Part model, mm, in its own coordinate system. Face numbers are marked on the shaded views. A direction names the side the tool comes from. Coordinates: 2 decimals unless noted, no trailing zeros. Order: outer loops, then holes, each group sorted by start corner. A loop starts at its lowest first (then second) coordinate and runs counter-clockwise, first axis right, second up. Notation, with made-up numbers: M 62,-28.5 L 117,-28.5 A19 ccw 117,4.5 Z; hole C 66.25,41.25 d3. An arc over 180 degrees is marked long. Answer in a Markdown table with one row per item. Add a question column.
from build123d import *

# Parameters (mm, degrees)
SKETCH1_W           = 30
SKETCH1_H           = 15
BOSS_EXTRUDE1_DEPTH = 15
SKETCH2_R           = 7.5
CUT_EXTRUDE1_DEPTH  = 15
CUT_EXTRUDE2_REACH  = 5
SKETCH3_R           = 2


with BuildPart() as part:
    # Sketch1 → Boss-Extrude1 (new body)
    with BuildSketch(Plane.XY):
        Rectangle(SKETCH1_W, SKETCH1_H)
    extrude(amount=BOSS_EXTRUDE1_DEPTH)

    # Sketch2 → Cut-Extrude1 (cut)
    with BuildSketch(Plane.XZ.offset(7.5)):
        with Locations((0, 15)):
            Circle(SKETCH2_R)
        with BuildLine():
            Line((-15, 12), (-9, 12))
            Line((-9, 12), (-8.485281374, 12))
            ThreePointArc((-8.485281374, 12), (0, 6), (8.485281374, 12))
            Line((8.485281374, 12), (9, 12))
            Line((9, 12), (15, 12))
            Line((15, 12), (15, 0))
            Line((15, 0), (11, 0))
            Line((11, 0), (-11, 0))
            Line((-11, 0), (-15, 0))
            Line((-15, 0), (-15, 12))
        make_face()
    extrude(amount=-CUT_EXTRUDE1_DEPTH, mode=Mode.SUBTRACT)

    # Sketch3 → Cut-Extrude2 (cut, up to next)
    with BuildSketch(Plane(origin=(0, 0, 12), x_dir=(-1, 0, 0), z_dir=(0, 0, -1)), mode=Mode.PRIVATE) as cut_extrude2_sk1:
        with Locations((11.3, -4.5)):
            Circle(SKETCH3_R)
    cut_extrude2_tool1 = extrude(cut_extrude2_sk1.sketch, amount=-CUT_EXTRUDE2_REACH, mode=Mode.PRIVATE) & part.part
    add(cut_extrude2_tool1.solids().sort_by_distance((-11.3, -4.5, 12))[0], mode=Mode.SUBTRACT)
    # Sketch3 → Cut-Extrude2 (cut, up to next)
    with BuildSketch(Plane(origin=(0, 0, 12), x_dir=(-1, 0, 0), z_dir=(0, 0, -1)), mode=Mode.PRIVATE) as cut_extrude2_sk2:
        with Locations((11.3, 4.5)):
            Circle(SKETCH3_R)
    cut_extrude2_tool2 = extrude(cut_extrude2_sk2.sketch, amount=-CUT_EXTRUDE2_REACH, mode=Mode.PRIVATE) & part.part
    add(cut_extrude2_tool2.solids().sort_by_distance((-11.3, 4.5, 12))[0], mode=Mode.SUBTRACT)
    # Sketch3 → Cut-Extrude2 (cut, up to next)
    with BuildSketch(Plane(origin=(0, 0, 12), x_dir=(-1, 0, 0), z_dir=(0, 0, -1)), mode=Mode.PRIVATE) as cut_extrude2_sk3:
        with Locations((-11.3, 4.5)):
            Circle(SKETCH3_R)
    cut_extrude2_tool3 = extrude(cut_extrude2_sk3.sketch, amount=-CUT_EXTRUDE2_REACH, mode=Mode.PRIVATE) & part.part
    add(cut_extrude2_tool3.solids().sort_by_distance((11.3, 4.5, 12))[0], mode=Mode.SUBTRACT)
    # Sketch3 → Cut-Extrude2 (cut, up to next)
    with BuildSketch(Plane(origin=(0, 0, 12), x_dir=(-1, 0, 0), z_dir=(0, 0, -1)), mode=Mode.PRIVATE) as cut_extrude2_sk4:
        with Locations((-11.3, -4.5)):
            Circle(SKETCH3_R)
    cut_extrude2_tool4 = extrude(cut_extrude2_sk4.sketch, amount=-CUT_EXTRUDE2_REACH, mode=Mode.PRIVATE) & part.part
    add(cut_extrude2_tool4.solids().sort_by_distance((11.3, -4.5, 12))[0], mode=Mode.SUBTRACT)


solid = part.part
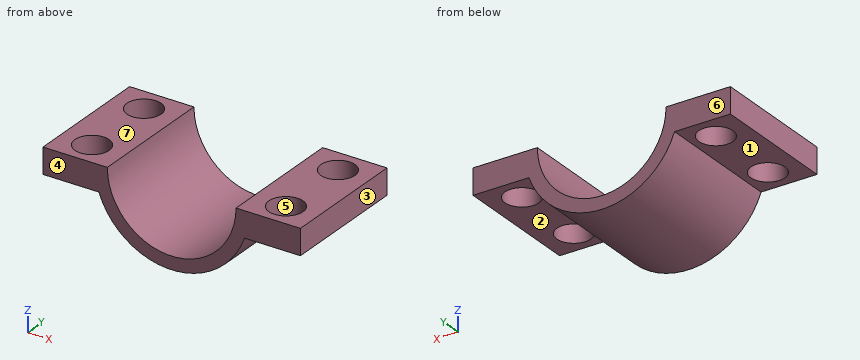
(1) Wall check: line 1 (Y direction, x = -11.3, z = 12.8); line 2 (Y direction, x = 10.25, z = 12.5); line 3 (X direction, y = -3, z = 12.5). Give the ranges that are in metal, low to high.
(2) Slice it at D-D (y = -1). List the corners of the cut face in (x, z).
(3) Drop flat-ended pins along their axis: P1, Ø4.5, axis at x = -11.3, y = 4.5, coming from the -Z side; P2, Ø1, axis at y = -2, z = 11, coming from the -X side; P3, Ø6.5, axis at x = -11.3, y = -4.5, coming from the -Z side. Give the stop position or say it passes through.
(4) 3-axis set-ups, long thin cutter, end or side, ignore diameter. For the marked faces 1, 2 and 3: which of +Z, -Z, +X, -X, +Y, -Y reach the whole face in a straight line?
(5) Slice it at A-A (x = -11.3). List the corners of the cut face in (y, z).
(6) Slice it at B-B (y = -4.5). List the corners of the cut face in (x, z), and give its area (3 significant figures).
(7) Pull direction Y, two halves, no side cores. Call the marked faces 4, 5, 6 and 7: pulls with the +Y half, pulls with the -Y half, needs draft (parallel to the pull), parting line crosses it, or undercut.
(8) Slice it at C-C (z = 8.5). List the corners of the cut face in (x, y), and give its area (3 significant figures).
Computed:
| question | item | result |
|---|---|---|
| 1 | line 1 | y = -7.5 to -6.5, -2.5 to 2.5, 6.5 to 7.5 |
| 1 | line 2 | y = -7.5 to -6.2, -2.8 to 2.8, 6.2 to 7.5 |
| 1 | line 3 | x = -15 to -12.62, -9.98 to -7.07, 7.07 to 9.98, 12.62 to 15 |
| 2 | outline | M -15,12 L -8.49,12 A9 ccw 8.49,12 L 15,12 L 15,15 L 7.5,15 A7.5 cw -7.5,15 L -15,15 Z |
| 3 | P1 | stops at z = 12 |
| 3 | P2 | stops at x = -8.29 |
| 3 | P3 | stops at z = 10.98 |
| 4 | face 1 | -Z, -X, +Y, -Y |
| 4 | face 2 | -Z, +X, +Y, -Y |
| 4 | face 3 | +Z, -Z, +X, +Y, -Y |
| 5 | outline | M -7.5,12 L -6.5,12 L -6.5,15 L -7.5,15 Z; M -2.5,12 L 2.5,12 L 2.5,15 L -2.5,15 Z; M 6.5,12 L 7.5,12 L 7.5,15 L 6.5,15 Z |
| 6 | outline | M -15,12 L -13.3,12 L -13.3,15 L -15,15 Z; M -9.3,12 L -8.49,12 A9 ccw 8.49,12 L 9.3,12 L 9.3,15 L 7.5,15 A7.5 cw -7.5,15 L -9.3,15 Z; M 13.3,12 L 15,12 L 15,15 L 13.3,15 Z |
| 6 | area | 51.9 mm^2 |
| 7 | face 4 | pulls with the -Y half |
| 7 | face 5 | undercut |
| 7 | face 6 | pulls with the +Y half |
| 7 | face 7 | needs draft |
| 8 | outline | M -6.22,-7.5 L -3.74,-7.5 L -3.74,7.5 L -6.22,7.5 Z; M 3.74,-7.5 L 6.22,-7.5 L 6.22,7.5 L 3.74,7.5 Z |
| 8 | area | 74.5 mm^2 |
